```python
from build123d import *

# Parameters (mm, degrees)
CROQUIS1_W              = 200
CROQUIS1_H              = 200
CROQUIS1_R              = 2.5
SALIENTE_EXTRUIR1_DEPTH = 4
CROQUIS2_W              = 158
CROQUIS2_H              = 158
CORTAR_EXTRUIR1_DEPTH   = 10
CROQUIS3_W              = 200
CROQUIS3_H              = 200
CROQUIS3_W_2            = 180
CROQUIS3_H_2            = 180
CORTAR_EXTRUIR2_DEPTH   = 10
CROQUIS4_W              = 158
CROQUIS4_H              = 5
CROQUIS4_W_2            = 5
CROQUIS4_H_2            = 158
CORTAR_EXTRUIR3_DEPTH   = 10


with BuildPart() as part:
    # Croquis1 → Saliente-Extruir1 (new body)
    with BuildSketch(Plane(origin=(0, 0, 0), x_dir=(1, 0, 0), z_dir=(0, 1, 0))):
        with Locations((100, 100)):
            Rectangle(CROQUIS1_W, CROQUIS1_H)
        with Locations(Location((15, 185, 0), (0, 0, 270))):
            Circle(CROQUIS1_R, mode=Mode.SUBTRACT)
        with Locations(Location((185, 185, 0), (0, 0, 270))):
            Circle(CROQUIS1_R, mode=Mode.SUBTRACT)
        with Locations(Location((185, 15, 0), (0, 0, 270))):
            Circle(CROQUIS1_R, mode=Mode.SUBTRACT)
        with Locations(Location((15, 15, 0), (0, 0, 270))):
            Circle(CROQUIS1_R, mode=Mode.SUBTRACT)
    extrude(amount=SALIENTE_EXTRUIR1_DEPTH)

    # Croquis2 → Cortar-Extruir1 (cut)
    with BuildSketch(Plane(origin=(0, 4, 0), x_dir=(1, 0, 0), z_dir=(0, 1, 0))):
        with Locations((100, 100)):
            Rectangle(CROQUIS2_W, CROQUIS2_H)
    extrude(amount=-CORTAR_EXTRUIR1_DEPTH, mode=Mode.SUBTRACT)

    # Croquis3 → Cortar-Extruir2 (cut)
    with BuildSketch(Plane(origin=(0, 4, 0), x_dir=(1, 0, 0), z_dir=(0, 1, 0))):
        with Locations((100, 100)):
            Rectangle(CROQUIS3_W, CROQUIS3_H)
        with Locations((100, 100)):
            Rectangle(CROQUIS3_W_2, CROQUIS3_H_2, mode=Mode.SUBTRACT)
    extrude(amount=-CORTAR_EXTRUIR2_DEPTH, mode=Mode.SUBTRACT)

    # Croquis4 → Cortar-Extruir3 (cut)
    with BuildSketch(Plane(origin=(0, 4, 0), x_dir=(1, 0, 0), z_dir=(0, 1, 0))):
        with Locations((100, 187.5)):
            Rectangle(CROQUIS4_W, CROQUIS4_H)
        with Locations((187.5, 100)):
            Rectangle(CROQUIS4_W_2, CROQUIS4_H_2)
        with Locations((100, 12.5)):
            Rectangle(CROQUIS4_W, CROQUIS4_H)
        with Locations((12.5, 100)):
            Rectangle(CROQUIS4_W_2, CROQUIS4_H_2)
    extrude(amount=-CORTAR_EXTRUIR3_DEPTH, mode=Mode.SUBTRACT)


solid = part.part
```
Geometry check sheet. Reference: the model listing, model coordinates, mm. A direction names the side the tool comes from. Coordinates: 2 decimals unless noted, no trailing zeros. Order: outer loops, then holes, each group sorted by start corner. A loop starts at its lowest first (then second) coordinate and runs counter-clockwise, first axis right, second up.
Item 1: Scan lines: line 1 along Z through (x, y) = (26.5, 3.6); line 2 along X through (y, z) = (0.2, -24). Record each from-to range of solid material in increasing order.
Item 2: Mould release check, pull along X, two halves, no side actions. Record for faces 1 (the flat face through (187, 2, -21)), 2 (the flat face through (190, 2, -15)), 3 (the flat face through (21, 2, -99)): released by +X, released by -X, zero draft, split by the parting line, or undercut.
Item 3: Section check C-C (y = 2.85). Enter the section's corners in (x, z).
Item 4: Tool access check on faces 4 (the flat face through (12, 2, -21)), 5 (the flat face through (179, 2, -12)), 6 (the flat face through (184, 2, -10)), 7 (the flat face through (179, 2, -187)), 8 (the flat face through (179, 2, -99)). Record the directions out of +Z, -Z, +X, -X, +Y, -Y that give a thin tool (end or side, any length) a straight path to the whole face; none if there is none.
Item 5: Section check A-A (z = -53.5). Enter the section's corners in (x, y), plus the area to 3 significant figures.
Item 6: Depth check by flat-ended pin: pin 1 (2 mm diameter, centred on x = 70, y = 3, fed in from -Z); pin 2 (2 mm diameter, centred on y = 2, z = -121, fed in from +X); pin 3 (1.2 mm diameter, centred on y = 1.5, z = -139, fed in from -X). Enter the tip coordinate at first touch or a pass-through.
Item 7: Section check B-B (x = 129.5). Enter the section's corners in (y, z), plus the area to 3 significant figures.
Check sheet entries:
1. line 1: z = -185 to -179, -21 to -15
1. line 2: x = 15 to 21, 179 to 185
2. face 1: zero draft
2. face 2: released by +X
2. face 3: undercut
3. outline: (10, -190) - (21, -190) - (21, -185) - (179, -185) - (179, -190) - (190, -190) - (190, -179) - (185, -179) - (185, -21) - (190, -21) - (190, -10) - (179, -10) - (179, -15) - (21, -15) - (21, -10) - (10, -10) - (10, -21) - (15, -21) - (15, -179) - (10, -179) - close; hole circle Ø5 at (15, -185); hole circle Ø5 at (15, -15); hole (21, -179) - (179, -179) - (179, -21) - (21, -21) - close; hole circle Ø5 at (185, -185); hole circle Ø5 at (185, -15)
4. face 4: -X, +Y, -Y
4. face 5: +Z, +Y, -Y
4. face 6: +Z, +X, -X, +Y, -Y
4. face 7: -Z, +Y, -Y
4. face 8: +Y, -Y
5. outline: (15, 0) - (21, 0) - (21, 4) - (15, 4) - close; (179, 0) - (185, 0) - (185, 4) - (179, 4) - close
5. area: 48.0 mm2
6. pin 1: stops at z = -185
6. pin 2: stops at x = 185
6. pin 3: stops at x = 15
7. outline: (0, -185) - (4, -185) - (4, -179) - (0, -179) - close; (0, -21) - (4, -21) - (4, -15) - (0, -15) - close
7. area: 48.0 mm2
